Build history of the part. All positions in model axes, mm. Round coordinates to 2 decimals unless told otherwise and drop trailing zeros. Write each loop counter-clockwise with the first axis right and the second up, starting at its lowest first coordinate (ties: lowest second). Pieces come first, ordered by that corner, then holes. Notation, with made-up numbers: M 43.25,49 L 101.25,49 A27 cw 101.25,72 Z; hole C 89,-20 d8. An arc over 180 degrees is marked long. Use a Markdown table: item, result.
from build123d import *

# Parameters (mm, degrees)
SKETCH1_W = 10
SKETCH1_H = 15


with BuildPart() as part:
    # Sketch1 → Revolve2 (revolve)
    with BuildSketch(Plane(origin=(0, 0, 0), x_dir=(0, 0, -1), z_dir=(1, 0, 0))):
        with BuildLine():
            Line((0, 25.4), (0, -25.4))
            ThreePointArc((0, -25.4), (-25.4, 0), (0, 25.4))
        make_face()
        with BuildLine():
            Line((0, -46.453146802), (0, -25.4))
            ThreePointArc((0, -25.4), (-6.051284035, -24.668643285), (-11.754091911, -22.516689884))
            Line((-11.754091911, -22.516689884), (-11.754091911, -25.953962773))
            add(Edge.make_bspline(
                [(-11.754091911, -25.953962773), (-13.625124372, -40.663791469), (-25.4, -39.846348213)],
                knots=[0, 0, 0, 1, 1, 1], degree=2))
            Line((-25.4, -39.846348213), (-25.4, -46.453146802))
            Line((-25.4, -46.453146802), (-10, -46.453146802))
            Line((-10, -46.453146802), (0, -46.453146802))
        make_face()
        with Locations((-5, -53.953146802)):
            Rectangle(SKETCH1_W, SKETCH1_H)
    revolve(axis=Axis((0, 38.955963628, 0), (0, -1, 0)))


solid = part.part
Q1. Drop flat-ended pins along their axis: P1, Ø4, axis at y = -38, z = 15, coming from the -X side; P2, Ø5, axis at x = 15, z = -1, coming from the +Y side; P3, Ø12, axis at x = 13, z = 16.5, coming from the -Y side. Give the stop position or say it passes through.
Response values:
| item | result |
|---|---|
| P1 | stops at x = -21.04 |
| P2 | stops at y = 22.09 |
| P3 | stops at y = -46.45 |
Q2. Drill centre lines: L1, parallel to Y at x = 10.5, z = 8.5; L2, parallel to Y at x = 14.5, z = -15.5; L3, parallel to Z at x = 1, y = -45.5. Where is each one in solid material? Low to high.
Response values:
| item | result |
|---|---|
| L1 | y = -46.45 to -32.82, -21.51 to 21.51 |
| L2 | y = -46.45 to -39.58, -13.95 to 13.95 |
| L3 | z = -25.38 to 25.38 |
Q3. Two-plate mould, pull along Y, no slides. Class faces 1 (the flat face through (0, -61.453, 0)), 2 (the cylindrical face through (24.796, -43.196, -5.506)), 3 (the cylindrical face through (-9.91, -24.26, 6.32)): +Y half, -Y half, draft (parallel to the pull), parting line (faces both ways), or undercut.
Response values:
| item | result |
|---|---|
| face 1 | -Y half |
| face 2 | draft |
| face 3 | undercut |
Q4. Cut at B-B on y = -3. Give the cut face in (x, z).
Response values:
| item | result |
|---|---|
| outline | C 0,0 d50.44 |
Q5. Cut at A-A on y = -48. Give the cut face in (x, z).
Response values:
| item | result |
|---|---|
| outline | C 0,0 d20 |
